Geometry check sheet. Reference: the model listing, model coordinates, mm. A direction names the side the tool comes from. Coordinates: 2 decimals unless noted, no trailing zeros. Write each loop counter-clockwise with the first axis right and the second up, starting at its lowest first coordinate (ties: lowest second). Pieces come first, ordered by that corner, then holes. Notation, with made-up numbers: (-30, 81.25) -> (14, 81.25) arc R27 cw to (14, 114.25) -> close; hole circle Ø4 at (53, 21). An arc over 180 degrees is marked (long way). Answer as CSV lines item,"result".
```python
from build123d import *

# Parameters (mm, degrees)
CROQUIS1_W                 = 42
CROQUIS1_H                 = 68
CROQUIS1_W_2               = 34
CROQUIS1_H_2               = 60
SALIENTE_EXTRUIR1_DEPTH    = 60
CROQUIS2_R                 = 2
CORTAR_EXTRUIR1_DEPTH      = 39
CORTAR_EXTRUIR1_DEPTH_BACK = 5
CROQUIS3_W                 = 42
CROQUIS3_H                 = 68
SALIENTE_EXTRUIR2_DEPTH    = 4
CROQUIS4_W                 = 64
CROQUIS4_H                 = 20
SALIENTE_EXTRUIR3_DEPTH    = 42
CROQUIS5_W                 = 42
CROQUIS5_H                 = 88
SALIENTE_EXTRUIR4_DEPTH    = 10
CROQUIS6_R                 = 1.2
CORTAR_EXTRUIR2_DEPTH      = 10


with BuildPart() as part:
    # Croquis1 → Saliente-Extruir1 (new body)
    with BuildSketch(Plane.XY):
        Rectangle(CROQUIS1_W, CROQUIS1_H)
        Rectangle(CROQUIS1_W_2, CROQUIS1_H_2, mode=Mode.SUBTRACT)
    extrude(amount=SALIENTE_EXTRUIR1_DEPTH)

    # Croquis2 → Cortar-Extruir1 (cut, two sides)
    with BuildSketch(Plane(origin=(-17, 0, 0), x_dir=(0, 0, -1), z_dir=(1, 0, 0))) as cortar_extruir1_sk:
        with Locations((-49.779, -10)):
            Circle(CROQUIS2_R)
        with Locations((-46.914797213, -3.085202787)):
            Circle(CROQUIS2_R)
        with Locations((-40, -0.221)):
            Circle(CROQUIS2_R)
        with Locations((-33.085202787, -3.085202787)):
            Circle(CROQUIS2_R)
        with Locations((-30.221, -10)):
            Circle(CROQUIS2_R)
        with Locations((-33.085202787, -16.914797213)):
            Circle(CROQUIS2_R)
        with Locations((-40, -19.779)):
            Circle(CROQUIS2_R)
        with Locations((-46.914797213, -16.914797213)):
            Circle(CROQUIS2_R)
    extrude(amount=CORTAR_EXTRUIR1_DEPTH, mode=Mode.SUBTRACT)
    extrude(cortar_extruir1_sk.sketch, amount=-CORTAR_EXTRUIR1_DEPTH_BACK, mode=Mode.SUBTRACT)

    # Croquis3 → Saliente-Extruir2 (add)
    with BuildSketch(Plane(origin=(0, 0, 0), x_dir=(-1, 0, 0), z_dir=(0, 0, -1))):
        Rectangle(CROQUIS3_W, CROQUIS3_H)
    extrude(amount=SALIENTE_EXTRUIR2_DEPTH)

    # Croquis4 → Saliente-Extruir3 (add)
    with BuildSketch(Plane(origin=(21, 0, 0), x_dir=(0, 0, -1), z_dir=(1, 0, 0))):
        with Locations((-28, -44)):
            Rectangle(CROQUIS4_W, CROQUIS4_H)
    extrude(amount=-SALIENTE_EXTRUIR3_DEPTH)

    # Croquis5 → Saliente-Extruir4 (add)
    with BuildSketch(Plane(origin=(0, 0, -4), x_dir=(-1, 0, 0), z_dir=(0, 0, -1))):
        with Locations((0, -10)):
            Rectangle(CROQUIS5_W, CROQUIS5_H)
    extrude(amount=SALIENTE_EXTRUIR4_DEPTH)

    # Croquis6 → Cortar-Extruir2 (cut)
    with BuildSketch(Plane(origin=(0, 0, -14), x_dir=(-1, 0, 0), z_dir=(0, 0, -1))):
        with Locations((0, -3)):
            Circle(CROQUIS6_R)
        with Locations((0, 8.6)):
            Circle(CROQUIS6_R)
        with Locations((7, -10)):
            Circle(CROQUIS6_R)
        with Locations((0, -17)):
            Circle(CROQUIS6_R)
        with Locations((-7, -10)):
            Circle(CROQUIS6_R)
        with Locations((0, -28.6)):
            Circle(CROQUIS6_R)
    extrude(amount=-CORTAR_EXTRUIR2_DEPTH, mode=Mode.SUBTRACT)


solid = part.part
```
Item 1: Thickness scan on probe 1 along Z at (x, y) = (18.65, -10); probe 2 along Y at (x, z) = (0, -7); probe 3 along X at (y, z) = (-26.5, 50.5). Record the ranges inside material, lowest first.
Responses:
probe 1,"z = -14 to 28.22, 32.22 to 47.78, 51.78 to 60"
probe 2,"y = -54 to -29.8, -27.4 to -18.2, -15.8 to -4.2, -1.8 to 7.4, 9.8 to 34"
probe 3,"x = -21 to -17, 17 to 21"
Item 2: Set-up check for faces 4 (the flat face through (17, 0, 30)), 5 (the flat face through (0, -17, -4)), 6 (the cylindrical face through (18.972, -2.997, 35.083)): record each of +Z, -Z, +X, -X, +Y, -Y from which the full face is reachable in a straight line by a thin tool's end or side.
Responses:
face 4,"+Z"
face 5,"-Z"
face 6,"+X, -X"
Item 3: Cross-section at D-D, the plane x = 4. Record the cut outline in (y, z), plus the area to 3 significant figures.
Responses:
outline,"(-54, -14) -> (34, -14) -> (34, 60) -> (30, 60) -> (30, 0) -> (-30, 0) -> (-30, 60) -> (-54, 60) -> close"
area,"2,910 mm2"
Item 4: Cross-section at C-C, the plane z = 4. Record the cut outline in (x, y).
Responses:
outline,"(-21, -54) -> (21, -54) -> (21, 34) -> (-21, 34) -> close; hole (-17, -30) -> (17, -30) -> (17, 30) -> (-17, 30) -> close"
Item 5: Depth check by flat-ended pin: pin 1 Ø2 at (x, y) = (0, 8.6) entering from +Z; pin 2 Ø1.9 at (x, y) = (-7, -10) entering from -Z; pin 3 Ø3.5 at (y, z) = (-10, 30.221) entering from -X. Enter the tip coordinate at first touch or a pass-through.
Responses:
pin 1,"stops at z = 0"
pin 2,"stops at z = -4"
pin 3,"passes through"
Item 6: Cross-section at B-B, the plane y = -10. Count the separate pieces of the cut face and the enclosed holes in it, plus the area to 3 significant figures.
Responses:
separate pieces,"5"
enclosed holes,"0"
area,"956 mm2"
Item 7: Release check for a two-part mould opening along Z. For faces 1 (the flat face through (-7, -10, -4)), 2 (the cylindrical face through (-0.554, -29.665, -9.07)), 3 (the cylindrical face through (-18.972, -0.133, 41.998)) record: +Z half, -Z half, draft (parallel to the pull), parting line (faces both ways), or undercut.
Responses:
face 1,"-Z half"
face 2,"draft"
face 3,"undercut"
Item 8: Cross-section at A-A, the plane z = 40. Record the cut outline in (x, y).
Responses:
outline,"(-21, -54) -> (21, -54) -> (21, -21.78) -> (17, -21.78) -> (17, -30) -> (-17, -30) -> (-17, -21.78) -> (-21, -21.78) -> close; (-21, -17.78) -> (-17, -17.78) -> (-17, -2.22) -> (-21, -2.22) -> close; (-21, 1.78) -> (-17, 1.78) -> (-17, 30) -> (17, 30) -> (17, 1.78) -> (21, 1.78) -> (21, 34) -> (-21, 34) -> close; (17, -17.78) -> (21, -17.78) -> (21, -2.22) -> (17, -2.22) -> close"
